from build123d import *

# Parameters (mm, degrees)
SKETCH_1_W          = 176
SKETCH_1_H          = 50
EXTRUDE_1_DEPTH     = 2
SKETCH_2_R          = 2.025
CUT_EXTRUDE_1_DEPTH = 22
CUT_EXTRUDE_2_DEPTH = 17
FILLET_1_R          = 2
SKETCH_4_R          = 2.025
CUT_EXTRUDE_3_DEPTH = 5
CUT_EXTRUDE_5_DEPTH = 15.5
SKETCH_8_W          = 22.857142857
SKETCH_8_H          = 30
CUT_EXTRUDE_6_DEPTH = 15.5
FILLET_2_R          = 2


with BuildPart() as part:
    # 草图1 → 凸台-拉伸1 (new, symmetric)
    with BuildSketch(Plane.XY):
        Rectangle(SKETCH_1_W, SKETCH_1_H)
    extrude(amount=EXTRUDE_1_DEPTH, both=True)

    # 草图2 → 切除-拉伸1 (cut, symmetric)
    with BuildSketch(Plane(origin=(0, 0, -2), x_dir=(-1, 0, 0), z_dir=(0, 0, -1))):
        with Locations((51.5, 21)):
            Circle(SKETCH_2_R)
        with Locations((51.5, -21)):
            Circle(SKETCH_2_R)
        with Locations((83.5, 21)):
            Circle(SKETCH_2_R)
        with Locations((83.5, -21)):
            Circle(SKETCH_2_R)
    cut_extrude_1 = extrude(amount=CUT_EXTRUDE_1_DEPTH, both=True, mode=Mode.SUBTRACT)

    # 镜向1: 切除-拉伸1 across plane
    add(cut_extrude_1.mirror(Plane(origin=(0, 0, 0), x_dir=(0, 0, 1), z_dir=(1, 0, 0))), mode=Mode.SUBTRACT)

    # 草图3 → 切除-拉伸2 (cut, symmetric)
    with BuildSketch(Plane(origin=(0, 0, -2), x_dir=(-1, 0, 0), z_dir=(0, 0, -1))):
        with BuildLine():
            Line((63.5, -21), (63.5, -25))
            Line((63.5, -25), (71.5, -25))
            Line((71.5, -25), (71.5, -21))
            ThreePointArc((71.5, -21), (67.5, -17), (63.5, -21))
        make_face()
    cut_extrude_2 = extrude(amount=CUT_EXTRUDE_2_DEPTH, both=True, mode=Mode.SUBTRACT)

    # 镜向2: 切除-拉伸2 across plane
    add(cut_extrude_2.mirror(Plane(origin=(0, 0, 0), x_dir=(0, 0, 1), z_dir=(1, 0, 0))), mode=Mode.SUBTRACT)

    # 圆角1
    fillet_1_edges = [part.edges().sort_by_distance(p)[0] for p in [
        (-71.5, -25, 0),
        (-63.5, -25, 0),
        (88, -25, 0),
        (-88, -25, 0),
        (-88, 25, 0),
        (88, 25, 0),
        (63.5, -25, 0),
        (71.5, -25, 0),
    ]]
    fillet(fillet_1_edges, radius=FILLET_1_R)

    # 草图4 → 切除-拉伸3 (cut, symmetric)
    with BuildSketch(Plane(origin=(0, 0, -2), x_dir=(-1, 0, 0), z_dir=(0, 0, -1))):
        with Locations((47.5, -12.5)):
            Circle(SKETCH_4_R)
        with Locations((47.5, 12.5)):
            Circle(SKETCH_4_R)
        with Locations((-47.5, 12.5)):
            Circle(SKETCH_4_R)
        with Locations((-47.5, -12.5)):
            Circle(SKETCH_4_R)
    extrude(amount=CUT_EXTRUDE_3_DEPTH, both=True, mode=Mode.SUBTRACT)

    # 草图7 → 切除-拉伸5 (cut, symmetric)
    with BuildSketch(Plane.XY.offset(2)):
        Polygon((-2, 19), (-45.032854639, 19), (-43.5, 15.742683893), (-43.5, -15.742683893), (-45.032854639, -19), (-2, -19), align=None)
        Polygon((45.032854639, 19), (2, 19), (2, -19), (45.032854639, -19), (43.5, -15.742683893), (43.5, 15.742683893), align=None)
    extrude(amount=CUT_EXTRUDE_5_DEPTH, both=True, mode=Mode.SUBTRACT)

    # 草图8 → 切除-拉伸6 (cut, symmetric)
    with BuildSketch(Plane.XY.offset(2)):
        with Locations((-69.023809524, 2)):
            Rectangle(SKETCH_8_W, SKETCH_8_H)
        with Locations((69.023809524, 2)):
            Rectangle(SKETCH_8_W, SKETCH_8_H)
    extrude(amount=CUT_EXTRUDE_6_DEPTH, both=True, mode=Mode.SUBTRACT)

    # 圆角2
    fillet_2_edges = [part.edges().sort_by_distance(p)[0] for p in [
        (-2, 19, 0),
        (-2, -19, 0),
        (-45.032854639, -19, 0),
        (-43.5, -15.742683893, 0),
        (-43.5, 15.742683893, 0),
        (-45.032854639, 19, 0),
        (2, 19, 0),
        (45.032854639, 19, 0),
        (43.5, 15.742683893, 0),
        (43.5, -15.742683893, 0),
        (45.032854639, -19, 0),
        (2, -19, 0),
        (-80.452380952, -13, 0),
        (-80.452380952, 17, 0),
        (-57.595238095, 17, 0),
        (-57.595238095, -13, 0),
        (80.452380952, 17, 0),
        (80.452380952, -13, 0),
        (57.595238095, -13, 0),
        (57.595238095, 17, 0),
    ]]
    fillet(fillet_2_edges, radius=FILLET_2_R)


solid = part.part
For this review, take the finished solid that the model builds, in its own axes (mm). A direction names the side the tool comes from. Give positions to 0.01 mm unless a question says otherwise; leave off trailing zeros. Loops run counter-clockwise (first coordinate to the right, second up) from the corner with the lowest first, then second, coordinate; pieces in that order, holes last. Notation, with made-up numbers: M 64,-10 L 108,-10 A26 ccw 108,18 Z; hole C 85,-18 d11. An arc over 180 degrees is marked long. Put each result on its own line as item: value. Start each with the question number.
(1) The part is to be moulded in two halves that separate along Y. For faces 3 (the flat face through (-69, -13, 0)), 4 (the flat face through (88, 0, 0)), 5 (the flat face through (-1, -25, 0)), say which applies: +Y half, -Y half, draft (parallel to the pull), parting line (faces both ways), or undercut.
(2) For pin 1 (1 mm diameter, centred on x = 42, y = -11, fed in from +Z), flat-tipped, find the tip position at first contact; note if it passes through.
(3) Wall thickness on L1, parallel to Y at x = 83.5, z = -0.15 (3 decimals); L2, parallel to X at y = 7, z = -0.5; L3, parallel to Y at x = 33, z = -0.55: over which ranges is each line inside the solid? List them lowest first.
(4) Add section D-D, the plane x = -23. Write out the cut boundary in (y, z), then the cut area to 3 significant figures.
(5) Add section A-A, the plane y = -4. Write out the cut boundary in (x, z), then the cut area to 3 significant figures.
(6) Add section B-B, the plane y = 12.5. Write out the cut boundary in (x, z) (3 decimals).
(7) Machinability: for faces 1 (the flat face through (-88, 0, 0)), 2 (the flat face through (-43.5, 0, 0)), which of the approach directions +Z, -Z, +X, -X, +Y, -Y give a long, thin tool a straight path to every point of the face, cutting with its end or side? Answer none if there is none.
(8) Add section C-C, the plane x = -51.5. Write out the cut boundary in (y, z) (3 decimals), then the cut area to 3 significant figures.
Result:
1. face 3: undercut
1. face 4: draft
1. face 5: -Y half
2. pin 1: passes through
3. L1: y = -25 to -23.025, -18.975 to 18.975, 23.025 to 25
3. L2: x = -88 to -80.45, -57.6 to -43.5, -2 to 2, 43.5 to 57.6, 80.45 to 88
3. L3: y = -25 to -19, 19 to 25
4. outline: M -25,-2 L -19,-2 L -19,2 L -25,2 Z; M 19,-2 L 25,-2 L 25,2 L 19,2 Z
4. area: 48.0 mm^2
5. outline: M -88,-2 L -80.45,-2 L -80.45,2 L -88,2 Z; M -57.6,-2 L -43.5,-2 L -43.5,2 L -57.6,2 Z; M -2,-2 L 2,-2 L 2,2 L -2,2 Z; M 43.5,-2 L 57.6,-2 L 57.6,2 L 43.5,2 Z; M 80.45,-2 L 88,-2 L 88,2 L 80.45,2 Z
5. area: 189 mm^2
6. outline: M -88,-2 L -80.452,-2 L -80.452,2 L -88,2 Z; M -57.595,-2 L -49.525,-2 L -49.525,2 L -57.595,2 Z; M -45.475,-2 L -43.5,-2 L -43.5,2 L -45.475,2 Z; M -2,-2 L 2,-2 L 2,2 L -2,2 Z; M 43.5,-2 L 45.475,-2 L 45.475,2 L 43.5,2 Z; M 49.525,-2 L 57.595,-2 L 57.595,2 L 49.525,2 Z; M 80.452,-2 L 88,-2 L 88,2 L 80.452,2 Z
7. face 1: +Z, -Z, -X, +Y, -Y
7. face 2: +Z, -Z
8. outline: M -25,-2 L -23.025,-2 L -23.025,2 L -25,2 Z; M -18.975,-2 L 18.975,-2 L 18.975,2 L -18.975,2 Z; M 23.025,-2 L 25,-2 L 25,2 L 23.025,2 Z
8. area: 168 mm^2
